```python
from build123d import *

# Parameters (mm, degrees)
CROQUIS3_R              = 16
SALIENTE_EXTRUIR2_DEPTH = 10
CROQUIS4_R              = 12
CORTAR_EXTRUIR1_DEPTH   = 10
ESCALA1_SCALE           = 7


with BuildPart() as part:
    # Croquis3 → Saliente-Extruir2 (new body)
    with BuildSketch(Plane.XY):
        Circle(CROQUIS3_R)
    extrude(amount=SALIENTE_EXTRUIR2_DEPTH)

    # Croquis4 → Cortar-Extruir1 (cut)
    with BuildSketch(Plane.XY.offset(10)):
        Circle(CROQUIS4_R)
    extrude(amount=-CORTAR_EXTRUIR1_DEPTH, mode=Mode.SUBTRACT)


with BuildPart() as part_1:
    # Escala1: scaled about (0, 0, 5)
    add(part.part.scale(ESCALA1_SCALE).moved(Location((0, 0, -30))))


solid = part_1.part
```
Work out the finished part from the listing and answer in its coordinate system (mm). Coordinates: 2 decimals unless noted, no trailing zeros. Loops run counter-clockwise (first coordinate to the right, second up) from the corner with the lowest first, then second, coordinate; pieces in that order, holes last. Notation, with made-up numbers: M 66.25,35.25 L 75.25,35.25 A6 ccw 75.25,42.25 Z; hole C -32,88.5 d11. An arc over 180 degrees is marked long. Use CSV: the item, a comma, the result in double quotes. Start each with the question number.
(1) Find section B-B, the plane y = 5. Give the vertices of the cut face in (x, z), then the cut area to 3 significant figures.
(2) Find section C-C, the plane z = 1.5. Give the vertices of the cut face in (x, y), then the cut area to 3 significant figures.
(3) Given pin 1 Ø8 at (y, z) = (71, 32.5) entering from -X; pin 2 Ø4 at (x, z) = (68, -4.5) entering from +Y; pin 3 Ø1 at (y, z) = (-7.5, 1) entering from -X, each flat-ended and moving along its own axis, determine where each tip first touches the part or whether it passes through.
(4) Consider line 1 (Y direction, x = 0, z = -7); line 2 (Y direction, x = -77, z = -7); line 3 (X direction, y = -67.5, z = 10). Determine where each line is inside the solid, lowest interval first.
(5) Find section A-A, the plane x = 0. Give the vertices of the cut face in (y, z).
(6) Find section D-D, the plane x = 89. Give the vertices of the cut face in (y, z).
(7) For a pull along X with two mould halves and no side action, classify faces 1 (the face through (80.12, 25.23, 5.49)), 2 (the face through (103.46, -42.9, 4.51)), 3 (the face through (16, 83, 40)) as +X half, -X half, draft (parallel to the pull), parting line (faces both ways), or undercut.
Recorded:
1,outline,"M -111.89,-30 L -83.85,-30 L -83.85,40 L -111.89,40 Z; M 83.85,-30 L 111.89,-30 L 111.89,40 L 83.85,40 Z"
1,area,"3,930 mm^2"
2,outline,"C 0,0 d224; hole C 0,0 d168"
2,area,"17,200 mm^2"
3,pin 1,"stops at x = -89.75"
3,pin 2,"stops at y = 90.49"
3,pin 3,"stops at x = -111.78"
4,line 1,"y = -112 to -84, 84 to 112"
4,line 2,"y = -81.33 to -33.57, 33.57 to 81.33"
4,line 3,"x = -89.37 to -50, 50 to 89.37"
5,outline,"M -112,-30 L -84,-30 L -84,40 L -112,40 Z; M 84,-30 L 112,-30 L 112,40 L 84,40 Z"
6,outline,"M -67.99,-30 L 67.99,-30 L 67.99,40 L -67.99,40 Z"
7,face 1,"undercut"
7,face 2,"parting line"
7,face 3,"draft"
